The model under review builds one solid part; all positions refer to its coordinate system, in mm. A direction names the side the tool comes from. Round coordinates to 2 decimals unless told otherwise and drop trailing zeros. Loops run counter-clockwise (first coordinate to the right, second up) from the corner with the lowest first, then second, coordinate; pieces in that order, holes last. Notation, with made-up numbers: M 59,21 L 84,21 A31 cw 84,47 Z; hole C 32,-40 d1. An arc over 180 degrees is marked long. Use a Markdown table: item, result. Add a question column.
```python
from build123d import *

# Parameters (mm, degrees)
SKETCH1_W           = 25.4
SKETCH1_H           = 25.4
SKETCH1_W_2         = 22.225
SKETCH1_H_2         = 22.225
BOSS_EXTRUDE1_DEPTH = 396.24
SKETCH3_R           = 2.54
CUT_EXTRUDE2_DEPTH  = 398.864873544
SKETCH4_R           = 2.54
CUT_EXTRUDE3_DEPTH  = 398.864873544


with BuildPart() as part:
    # Sketch1 → Boss-Extrude1 (new body)
    with BuildSketch(Plane.XY):
        with Locations((12.7, 12.7)):
            Rectangle(SKETCH1_W, SKETCH1_H)
        with Locations((12.7, 12.7)):
            Rectangle(SKETCH1_W_2, SKETCH1_H_2, mode=Mode.SUBTRACT)
    extrude(amount=BOSS_EXTRUDE1_DEPTH)

    # Sketch3 → Cut-Extrude2 (cut, through all)
    with BuildSketch(Plane(origin=(0, 25.4, 0), x_dir=(1, 0, 0), z_dir=(0, 1, 0))):
        with Locations(Location((15.875, -383.54, 0), (0, 0, 270))):
            Circle(SKETCH3_R)
        with Locations(Location((15.875, -12.7, 0), (0, 0, 270))):
            Circle(SKETCH3_R)
    extrude(amount=-CUT_EXTRUDE2_DEPTH, mode=Mode.SUBTRACT)

    # Sketch4 → Cut-Extrude3 (cut, through all)
    with BuildSketch(Plane(origin=(25.4, 0, 0), x_dir=(0, 0, -1), z_dir=(1, 0, 0))):
        with Locations((-383.54, 12.7)):
            Circle(SKETCH4_R)
        with Locations((-358.14, 12.7)):
            Circle(SKETCH4_R)
        with Locations((-332.74, 12.7)):
            Circle(SKETCH4_R)
        with Locations((-307.34, 12.7)):
            Circle(SKETCH4_R)
        with Locations((-281.94, 12.7)):
            Circle(SKETCH4_R)
        with Locations((-256.54, 12.7)):
            Circle(SKETCH4_R)
        with Locations((-231.14, 12.7)):
            Circle(SKETCH4_R)
        with Locations(Location((-165.1, 12.7, 0), (0, 0, 180))):
            Circle(SKETCH4_R)
        with Locations(Location((-139.7, 12.7, 0), (0, 0, 180))):
            Circle(SKETCH4_R)
        with Locations(Location((-114.3, 12.7, 0), (0, 0, 180))):
            Circle(SKETCH4_R)
        with Locations(Location((-88.9, 12.7, 0), (0, 0, 180))):
            Circle(SKETCH4_R)
        with Locations(Location((-63.5, 12.7, 0), (0, 0, 180))):
            Circle(SKETCH4_R)
        with Locations(Location((-38.1, 12.7, 0), (0, 0, 180))):
            Circle(SKETCH4_R)
        with Locations(Location((-12.7, 12.7, 0), (0, 0, 180))):
            Circle(SKETCH4_R)
    extrude(amount=-CUT_EXTRUDE3_DEPTH, mode=Mode.SUBTRACT)


solid = part.part
```
(1) To check wall thickness, follow probe 1 along Y at (x, z) = (2, 209.5); probe 2 along Y at (x, z) = (24.2, 231.14). State the ranges of each line that lie inside material, in increasing order.
(2) For faces 1 (the face through (1, 13, 396.24)), 2 (the face through (23.812, 13, 195)), list the 3-axis set-ups (+Z, -Z, +X, -X, +Y, -Y) from which the entire face can be reached by the end or side of a thin tool; tool diameter is ignored.
(3) Draft analysis for pull direction X (two halves, no side actions). For faces 3 (the face through (25.4, 13, 195)), 4 (the face through (0, 13, 195)), 5 (the face through (13, 23.812, 195)), 6 (the face through (13, 1.587, 195)), state which applies: released by +X, released by -X, zero draft, split by the parting line, or undercut.
(4) Consider section A-A, the plane z = 289. Give the boundary of the cut face in (x, y), then the cut area to 3 significant figures.
Found:
| question | item | result |
|---|---|---|
| 1 | probe 1 | y = 0 to 1.59, 23.81 to 25.4 |
| 1 | probe 2 | y = 0 to 10.16, 15.24 to 25.4 |
| 2 | face 1 | +Z, +X, -X, +Y, -Y |
| 2 | face 2 | +Z, -Z |
| 3 | face 3 | released by +X |
| 3 | face 4 | released by -X |
| 3 | face 5 | undercut |
| 3 | face 6 | undercut |
| 4 | outline | M 0,0 L 25.4,0 L 25.4,25.4 L 0,25.4 Z; hole M 1.59,1.59 L 23.81,1.59 L 23.81,23.81 L 1.59,23.81 Z |
| 4 | area | 151 mm^2 |
